Source: CAD feature listing. Evaluate the final solid. Frame: model axes, mm. Face numbers are marked on the shaded views. A direction names the side the tool comes from. Round coordinates to 2 decimals unless told otherwise and drop trailing zeros. Write each loop counter-clockwise with the first axis right and the second up, starting at its lowest first coordinate (ties: lowest second). Pieces come first, ordered by that corner, then holes. Notation, with made-up numbers: M 85,43.5 L 109,43.5 A24 ccw 109,68.5 Z; hole C 77.25,-3.75 d9. An arc over 180 degrees is marked long. Answer in a Markdown table with one row per item. Add a question column.
Item 1: Cut plane A-A on x = 12. Return loops of the section in (y, z), and give its area (3 significant figures).
Item 2: Set-up query: the marked faces 1 and 2. Return all of +Z, -Z, +X, -X, +Y, -Y with unobstructed straight access to the full face (end or side cutting, diameter ignored); none if empty.
Item 3: Mould query, pull axis X, two halves, no side actions, for the marked faces 3, 4 and 5. Classes: released by +X, released by -X, zero draft, split by the parting line, or undercut.
Item 4: Contact query for flat-ended pins moving along their axis: pin 1 (1 mm diameter, centred on y = -3.5, z = 5.5, fed in from +X); pin 2 (2.5 mm diameter, centred on x = 12, z = -2.5, fed in from +Y); pin 3 (2 mm diameter, centred on x = 10, z = 7.5, fed in from -Y). Output: stop coordinate, or through.
Item 5: Cut plane C-C on y = -2.55. Return loops of the section in (x, z), and give its area (3 significant figures).
Item 6: Cut plane D-D on x = -5. Return loops of the section in (y, z), and give its area (3 significant figures).
Item 7: Material intervals for probe 1 along Z at (x, y) = (12, -3.05); probe 2 along Z at (x, y) = (-12, -2.4); probe 3 along X at (y, z) = (-0.9, -1.5), sorted ascending.
Item 8: Cut plane B-B on z = -2.5. Return loops of the section in (x, y), and give its area (3 significant figures).
from build123d import *

# Parameters (mm, degrees)
F0_W           = 30
F0_H           = 7.5
F1_DEPTH       = 2
F0_W_2         = 10
F2_DEPTH       = 4
F3_D           = 3.3
F3_CSINK_D     = 6.72
F3_CSINK_ANGLE = 90
F4_R           = 5


with BuildPart() as f1:
    # F0 (on Front) → F1 (new body)
    with BuildSketch(Plane.XZ):
        with Locations((5, 6.25)):
            Rectangle(F0_W, F0_H)
    extrude(amount=F1_DEPTH)

    # F0 (on Front) → F2 (join)
    with BuildSketch(Plane.XZ):
        Polygon((-20, -10), (20, -10), (20, 2.5), (-10, 2.5), (-20, 2.5), align=None)
        with Locations((-15, 6.25)):
            Rectangle(F0_W_2, F0_H)
    extrude(amount=F2_DEPTH)

    # F3 (through all)
    with Locations(Plane(origin=(0, 0, 0), x_dir=(1, 0, 0), z_dir=(0, 1, 0))):
        with Locations((-12, 2.5), (12, 2.5)):
            CounterSinkHole(F3_D / 2, F3_CSINK_D / 2, counter_sink_angle=F3_CSINK_ANGLE)

    # F4
    f4_edges = [f1.edges().sort_by_distance(p)[0] for p in [
        (-20, -2, -10),
    ]]
    fillet(f4_edges, radius=F4_R)


solid = f1.part
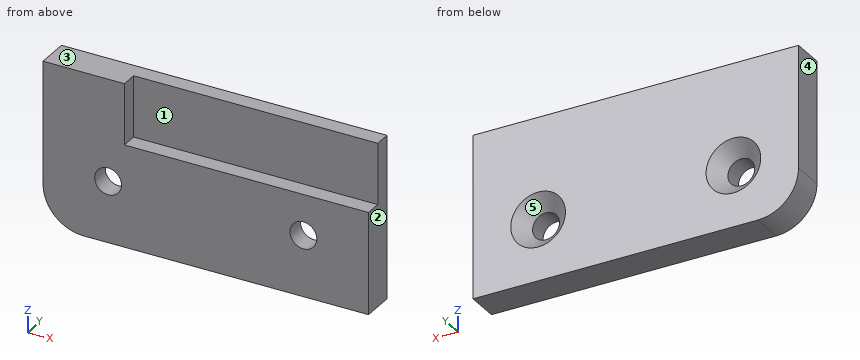
Results below:
| question | item | result |
|---|---|---|
| 1 | outline | M -4,-10 L 0,-10 L 0,-5.86 L -1.71,-4.15 L -4,-4.15 Z; M -4,-0.85 L -1.71,-0.85 L 0,0.86 L 0,10 L -2,10 L -2,2.5 L -4,2.5 Z |
| 1 | area | 48.9 mm2 |
| 2 | face 1 | +Z, +X, -Y |
| 2 | face 2 | +Z, -Z, +X, +Y, -Y |
| 3 | face 3 | zero draft |
| 3 | face 4 | released by -X |
| 3 | face 5 | undercut |
| 4 | pin 1 | x = -10 |
| 4 | pin 2 | through |
| 4 | pin 3 | y = -2 |
| 5 | outline | M -20,-5 A5 ccw -15,-10 L 20,-10 L 20,2.5 L -10,2.5 L -10,10 L -20,10 Z; hole C -12,-2.5 d3.3; hole C 12,-2.5 d3.3 |
| 5 | area | 553 mm2 |
| 6 | outline | M -4,-10 L 0,-10 L 0,10 L -2,10 L -2,2.5 L -4,2.5 Z |
| 6 | area | 65.0 mm2 |
| 7 | probe 1 | -10 to -4.15, -0.85 to 2.5 |
| 7 | probe 2 | -10 to -4.15, -0.85 to 10 |
| 7 | probe 3 | -20 to -14.25, -9.75 to 9.75, 14.25 to 20 |
| 8 | outline | M -20,-4 L -13.65,-4 L -13.65,-1.71 L -15.36,0 L -20,0 Z; M -10.35,-4 L 10.35,-4 L 10.35,-1.71 L 8.64,0 L -8.64,0 L -10.35,-1.71 Z; M 13.65,-4 L 20,-4 L 20,0 L 15.36,0 L 13.65,-1.71 Z |
| 8 | area | 128 mm2 |
